Could you check a few things on this model? Use its own coordinates, in mm. A direction names the side the tool comes from. Round coordinates to 2 decimals unless told otherwise and drop trailing zeros. Write each loop counter-clockwise with the first axis right and the second up, starting at its lowest first coordinate (ties: lowest second). Pieces come first, ordered by that corner, then holes. Notation, with made-up numbers: (63.5, 7) -> (111.5, 7) arc R17 cw to (111.5, 27) -> close; hole circle Ø6 at (14.5, 54.5). An arc over 180 degrees is marked (long way). One line per question, with ' | ' between items. Start each with the question number.
1. Imagine slicing it at A-A, the plane x = -27. List the corners of the cut face in (y, z) for me.
2. For pin 1 Ø4 at (x, y) = (13.5, 3) entering from -Z; pin 2 Ø1.9 at (x, z) = (0.5, 46) entering from -Y; pin 3 Ø2 at (x, y) = (-8.5, 11) entering from -Z, each with a flat end and sliding along its axis, tell me the tip position at first contact or that it passes through.
3. Imagine slicing it at B-B, the plane y = -28. List the corners of the cut face in (x, z) for me.
4. For faces 1 (the flat face through (-29.855, 5.134, 5.303)), 2 (the flat face through (-29.2, 5.134, -5.454)), 3 (the flat face through (0, 0, -43)), which set-ups out of +Z, -Z, +X, -X, +Y, -Y let a thin tool reach every point of the face, with its end or its side?
5. Imagine slicing it at D-D, the plane x = 44.5. List the corners of the cut face in (y, z) for me, and give its area (3 significant figures).
6. Imagine slicing it at C-C, the plane z = 9. List the corners of the cut face in (x, y) for me.
7. If I drill on line 1 along Y through (x, z) = (-24.5, 7); line 2 along Y through (x, z) = (25.5, 4); line 3 along Z through (x, y) = (1, 28), over which ranges is the centre line in solid material (lowest first)? Write a range as [from, to].
from build123d import *

# Parameters (mm, degrees)
F0_R     = 33.795708
F1_DEPTH = 18.288
F2_R     = 5.368013
F3_DEPTH = 47.498
F4_R     = 5.08
F5_R     = 5.839733
F6_DEPTH = 34.544
F7_W     = 12.265376
F7_H     = 21.514286
F8_DEPTH = 10.414


with BuildPart() as f1:
    # F0 (on Front) → F1 (new body)
    with BuildSketch(Plane.XZ):
        Circle(F0_R)
    extrude(amount=F1_DEPTH)

    # F2 (on face) → F3 (join)
    with BuildSketch(Plane.XZ.offset(18.288)):
        Circle(F2_R)
    extrude(amount=F3_DEPTH)

    # F4
    f4_edges = [f1.edges().sort_by_distance(p)[0] for p in [
        (-5.368013, -65.786, 0),
    ]]
    fillet(f4_edges, radius=F4_R)

    # F5 (on face) → F6 (join)
    with BuildSketch(Plane(origin=(0, 0, 0), x_dir=(-1, 0, 0), z_dir=(0, 1, 0))):
        Circle(F5_R)
    extrude(amount=F6_DEPTH)

    # F7 (on face) → F8 (join)
    with BuildSketch(Plane(origin=(0, 0, 0), x_dir=(-1, 0, 0), z_dir=(0, 1, 0))):
        Polygon((-52.923243, 0), (-6.132688, -10.757143), (-6.132688, 10.757143), align=None)
        Polygon((6.132688, -10.757143), (-6.132688, -10.757143), (0, -58.2073), (6.389142, -10.757143), align=None)
        Rectangle(F7_W, F7_H)
        Polygon((6.132688, 10.757143), (6.132688, -10.757143), (52.923243, 0), align=None)
        Polygon((0, 58.2073), (-6.132688, 10.757143), (6.132688, 10.757143), (6.389142, 10.757143), align=None)
    extrude(amount=F8_DEPTH)


solid = f1.part
Geometry results:
1) outline: (-18.29, -20.33) -> (0, -20.33) -> (0, -5.96) -> (10.41, -5.96) -> (10.41, 5.96) -> (0, 5.96) -> (0, 20.33) -> (-18.29, 20.33) -> close
2) pin 1: stops at z = -9.52 | pin 2: stops at y = 0 | pin 3: stops at z = -10.4
3) outline: circle Ø10.74 at (0, 0)
4) face 1: +Z, -X, +Y | face 2: -Z, -X, +Y | face 3: -Z, +X, -X, -Y
5) outline: (0, -1.94) -> (10.41, -1.94) -> (10.41, 1.94) -> (0, 1.94) -> close | area: 40.3 mm2
6) outline: (-32.58, -18.29) -> (32.58, -18.29) -> (32.58, 0) -> (13.78, 0) -> (13.78, 10.41) -> (-13.78, 10.41) -> (-13.78, 0) -> (-32.58, 0) -> close
7) line 1: y = [-18.29, 0] | line 2: y = [-18.29, 10.41] | line 3: z = [-5.75, 5.75]
